from build123d import *

# Parameters (mm, degrees)
ESQUISSE1_R        = 20.5
BOSS_EXTRU_1_DEPTH = 2
ESQUISSE2_R        = 2
GOUJON_M4X10_DEPTH = 10
ESQUISSE3_R        = 2
GOUJON_M4X20_DEPTH = 20


with BuildPart() as part:
    # Esquisse1 → Boss.-Extru.1 (new body)
    with BuildSketch(Plane.XY):
        with BuildLine():
            Line((-90, -160), (90, -160))
            Line((90, -160), (90, 0))
            ThreePointArc((90, 0), (0, 90), (-90, 0))
            Line((-90, 0), (-90, -160))
        make_face()
        Circle(ESQUISSE1_R, mode=Mode.SUBTRACT)
    extrude(amount=BOSS_EXTRU_1_DEPTH)

    # Esquisse2 → Goujon M4x10 (add)
    with BuildSketch(Plane.XY.offset(2)):
        with Locations((-17.67766953, 17.67766953)):
            Circle(ESQUISSE2_R)
        with Locations((17.67766953, 17.67766953)):
            Circle(ESQUISSE2_R)
        with Locations((17.67766953, -17.67766953)):
            Circle(ESQUISSE2_R)
        with Locations((-17.67766953, -17.67766953)):
            Circle(ESQUISSE2_R)
    extrude(amount=GOUJON_M4X10_DEPTH)

    # Esquisse3 → Goujon M4x20 (add)
    with BuildSketch(Plane.XY.offset(2)):
        with Locations((-20, -100)):
            Circle(ESQUISSE3_R)
        with Locations((20, -100)):
            Circle(ESQUISSE3_R)
    extrude(amount=GOUJON_M4X20_DEPTH)


solid = part.part
Geometry check sheet. Reference: the model listing, model coordinates, mm. Give positions to 0.01 mm unless a question says otherwise; leave off trailing zeros. Write each loop counter-clockwise with the first axis right and the second up, starting at its lowest first coordinate (ties: lowest second). Pieces come first, ordered by that corner, then holes. Notation, with made-up numbers: M 13,-26 L 49,-26 A27 ccw 49,6 Z; hole C -36,50 d9. An arc over 180 degrees is marked long. One line per question, with ' | ' between items.
1. Cross-section at C-C (z = 17.25). Enter the section's corners in (x, y).
Ans:
outline: C -20,-100 d4; C 20,-100 d4
2. Cross-section at B-B (y = 13). Enter the section's corners in (x, z), plus the area to 3 significant figures.
Ans:
outline: M -89.06,0 L -15.85,0 L -15.85,2 L -89.06,2 Z; M 15.85,0 L 89.06,0 L 89.06,2 L 15.85,2 Z | area: 293 mm2
3. Cross-section at A-A (x = 0). Enter the section's corners in (y, z).
Ans:
outline: M -160,0 L -20.5,0 L -20.5,2 L -160,2 Z; M 20.5,0 L 90,0 L 90,2 L 20.5,2 Z
4. Cross-section at D-D (y = -52). Enter the section's corners in (x, z).
Ans:
outline: M -90,0 L 90,0 L 90,2 L -90,2 Z
5. Scan lines: line 1 along Y through (x, z) = (0, 1.1); line 2 along Z through (x, y) = (-1, -64); line 3 along Y through (x, z) = (-42.5, 1.5). Record each from-to range of solid material in increasing order. Write a range as from..to.
Ans:
line 1: -160..-20.5, 20.5..90 | line 2: 0..2 | line 3: -160..79.33
6. Mould release check, pull along X, two halves, no side actions. Record for faces 1 (the face through (-4.444, -20.013, 0.986)), 2 (the face through (1.98, 89.98, 0.99)), 3 (the face through (-1, -33, 0)): released by +X, released by -X, zero draft, split by the parting line, or undercut.
Ans:
face 1: undercut | face 2: split by the parting line | face 3: zero draft
7. Gauge pin test, flat ends, axial feed: pin 1 (12 mm diameter, centred on x = -23.5, z = 12.5, fed in from -Y); pin 2 (10 mm diameter, centred on y = 18.5, z = 9, fed in from -X); pin 3 (3 mm diameter, centred on x = -17.5, y = 17.5, fed in from +Z). Record the tip position at first contact, or that the pin passes through.
Ans:
pin 1: y = -102 | pin 2: x = -19.68 | pin 3: z = 12
